from build123d import *

# Parameters (mm, degrees)
SKETCH1_R             = 2
SKETCH1_R_2           = 1.25
BOSS_EXTRUDE1_DEPTH   = 6.1
BOSS_EXTRUDE1_2_DEPTH = 6.1
BOSS_EXTRUDE1_3_DEPTH = 6.1
BOSS_EXTRUDE2_DEPTH   = 1
CUT_EXTRUDE1_REACH    = 18.114
SKETCH6_R             = 1.25


with BuildPart() as part:
    # Sketch1 → Boss-Extrude1 (new body)
    with BuildSketch(Plane.XY):
        with Locations((4, 3.947606604)):
            Circle(SKETCH1_R)
        with Locations((4, 3.947606604)):
            Circle(SKETCH1_R_2, mode=Mode.SUBTRACT)
    extrude(amount=BOSS_EXTRUDE1_DEPTH)



with BuildPart() as body_2:
    # Sketch1 → Boss-Extrude1 2 (new body)
    with BuildSketch(Plane.XY):
        with Locations(Location((-4, 3.947606604, 0), (0, 0, 180))):
            Circle(SKETCH1_R)
        with Locations(Location((-4, 3.947606604, 0), (0, 0, 180))):
            Circle(SKETCH1_R_2, mode=Mode.SUBTRACT)
    extrude(amount=BOSS_EXTRUDE1_2_DEPTH)


with BuildPart() as body_3:
    # Sketch1 → Boss-Extrude1 3 (new body)
    with BuildSketch(Plane.XY):
        with BuildLine():
            Line((7.350565553, 4.525283395), (10.814667168, 6.525283395))
            Line((10.814667168, 6.525283395), (11.414667168, 5.486052911))
            Line((11.414667168, 5.486052911), (8.599175725, 3.860528168))
            ThreePointArc((8.599175725, 3.860528168), (5.132583975, -0.510784758), (0, 1.676043266))
            ThreePointArc((0, 1.676043266), (-5.132583975, -0.510784758), (-8.599175725, 3.860528168))
            Line((-8.599175725, 3.860528168), (-11.414667168, 5.486052911))
            Line((-11.414667168, 5.486052911), (-10.814667168, 6.525283395))
            Line((-10.814667168, 6.525283395), (-7.350565553, 4.525283395))
            ThreePointArc((-7.350565553, 4.525283395), (-1.055513627, 2.247606604), (-6.175565553, 6.560443094))
            Line((-6.175565553, 6.560443094), (-9.639667168, 8.560443094))
            Line((-9.639667168, 8.560443094), (-9.039667168, 9.599673579))
            Line((-9.039667168, 9.599673579), (-6.224175725, 7.974148836))
            ThreePointArc((-6.224175725, 7.974148836), (-2.751650813, 8.374978771), (0, 6.219169942))
            ThreePointArc((0, 6.219169942), (2.751650813, 8.374978771), (6.224175725, 7.974148836))
            Line((6.224175725, 7.974148836), (9.039667168, 9.599673579))
            Line((9.039667168, 9.599673579), (9.639667168, 8.560443094))
            Line((9.639667168, 8.560443094), (6.175565553, 6.560443094))
            ThreePointArc((6.175565553, 6.560443094), (1.055513627, 2.247606604), (7.350565553, 4.525283395))
        make_face()
    extrude(amount=BOSS_EXTRUDE1_3_DEPTH)


with BuildPart() as part_1:
    add(part.part)

    add(body_2.part)  # Boss-Extrude2 merges body 2

    add(body_3.part)  # Boss-Extrude2 merges body 3
    # Sketch2 → Boss-Extrude2 (add)
    with BuildSketch(Plane(origin=(0, 0, 0), x_dir=(-1, 0, 0), z_dir=(0, 0, -1))):
        with BuildLine():
            Line((-9.639667168, 8.560443094), (-10.814667168, 6.525283395))
            Line((-10.814667168, 6.525283395), (-11.414667168, 5.486052911))
            Line((-11.414667168, 5.486052911), (-8.599175725, 3.860528168))
            ThreePointArc((-8.599175725, 3.860528168), (-5.132583975, -0.510784758), (0, 1.676043266))
            ThreePointArc((0, 1.676043266), (5.132583975, -0.510784758), (8.599175725, 3.860528168))
            Line((8.599175725, 3.860528168), (11.414667168, 5.486052911))
            Line((11.414667168, 5.486052911), (10.814667168, 6.525283395))
            Line((10.814667168, 6.525283395), (9.639667168, 8.560443094))
            Line((9.639667168, 8.560443094), (9.039667168, 9.599673579))
            Line((9.039667168, 9.599673579), (6.224175725, 7.974148836))
            ThreePointArc((6.224175725, 7.974148836), (2.751650813, 8.374978771), (0, 6.219169942))
            ThreePointArc((0, 6.219169942), (-2.751650813, 8.374978771), (-6.224175725, 7.974148836))
            Line((-6.224175725, 7.974148836), (-9.039667168, 9.599673579))
            Line((-9.039667168, 9.599673579), (-9.639667168, 8.560443094))
        make_face()
    extrude(amount=BOSS_EXTRUDE2_DEPTH)

    # Sketch6 → Cut-Extrude1 (cut, up to next)
    with BuildSketch(Plane.XY, mode=Mode.PRIVATE) as cut_extrude1_sk1:
        with Locations(Location((4, 3.947606604, 0), (0, 0, 180))):
            Circle(SKETCH6_R)
    cut_extrude1_tool1 = extrude(cut_extrude1_sk1.sketch, amount=-CUT_EXTRUDE1_REACH, mode=Mode.PRIVATE) & part_1.part
    # Sketch6 → Cut-Extrude1 (cut, up to next)
    with BuildSketch(Plane.XY, mode=Mode.PRIVATE) as cut_extrude1_sk2:
        with Locations(Location((-4, 3.947606604, 0), (0, 0, 180))):
            Circle(SKETCH6_R)
    cut_extrude1_tool2 = extrude(cut_extrude1_sk2.sketch, amount=-CUT_EXTRUDE1_REACH, mode=Mode.PRIVATE) & part_1.part
    add(cut_extrude1_tool1.solids().sort_by_distance((4, 3.947607, 0))[0], mode=Mode.SUBTRACT)
    add(cut_extrude1_tool2.solids().sort_by_distance((-4, 3.947607, 0))[0], mode=Mode.SUBTRACT)


solid = part_1.part
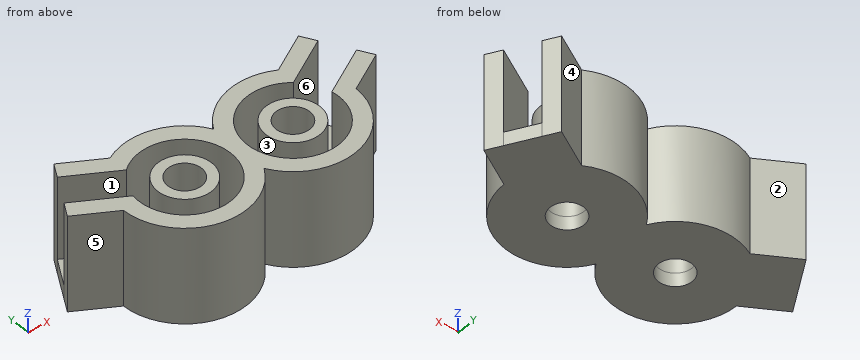
Design review of the part built by this model. Coordinates are the model's own, in mm. Face numbers are marked on the shaded views. A direction names the side the tool comes from. Give positions to 0.01 mm unless a question says otherwise; leave off trailing zeros. Write each loop counter-clockwise with the first axis right and the second up, starting at its lowest first coordinate (ties: lowest second). Pieces come first, ordered by that corner, then holes. Notation, with made-up numbers: M 30,23.5 L 46,23.5 A36 cw 46,57.5 Z; hole C 66.25,26.25 d1. An arc over 180 degrees is marked long. Answer as a JSON object with one key per item and string values. Group by question number.
1) Clearance check with flat-ended pins moving along their axes: pin 1 Ø1.5 at (y, z) = (5.5, 0.5) entering from +X; pin 2 Ø4 at (x, z) = (8, 5) entering from +Y; pin 3 Ø3 at (x, z) = (-7, 3) entering from +Y; pin 4 Ø1 at (x, z) = (7.5, 2.5) entering from +Y. State where each tip first meets the part, or that it passes through.
2) Mouldability with a two-part tool opening along Y and no side actions: class the marked faces 4, 5 and 6 as released by +Y, released by -Y, zero draft, split by the parting line, or undercut.
3) For line 1 along Y through (x, z) = (4, 3); line 2 along X through (y, z) = (1.75, 4); line 3 along Y through (x, z) = (-4, -0.5), list the stretches that pass through material, from the lowest coordinate up.
4) We need section A-A (x = -4). Give the boundary of the cut face in (y, z), and give its area (3 significant figures).
5) Tool access review of the marked faces 1, 2 and 3: name each direction out of +Z, -Z, +X, -X, +Y, -Y from which nothing blocks a thin tool from reaching the whole face with its end or side.
6) We need section B-B (x = -8). Give the boundary of the cut face in (y, z).
Answer key:
{
 "1": {"pin 1": "stops at x = 11.41", "pin 2": "stops at y = 9.6", "pin 3": "stops at y = 9.29", "pin 4": "stops at y = 9"},
 "2": {"face 4": "released by +Y", "face 5": "released by -Y", "face 6": "undercut"},
 "3": {"line 1": "y = -0.65 to 0.55, 1.95 to 2.7, 5.2 to 5.95, 7.35 to 8.55", "line 2": "x = -8.04 to -6.59, -1.41 to 1.41, 6.59 to 8.04", "line 3": "y = -0.65 to 2.7, 5.2 to 8.55"},
 "4": {"outline": "M -0.65,-1 L 2.7,-1 L 2.7,6.1 L 1.95,6.1 L 1.95,0 L 0.55,0 L 0.55,6.1 L -0.65,6.1 Z; M 5.2,-1 L 8.55,-1 L 8.55,6.1 L 7.35,6.1 L 7.35,0 L 5.95,0 L 5.95,6.1 L 5.2,6.1 Z", "area": "30.5 mm²"},
 "5": {"face 1": "+Z, -X", "face 2": "+Z, -Z, +Y", "face 3": "+Z"},
 "6": {"outline": "M 1.68,-1 L 9,-1 L 9,6.1 L 7.61,6.1 L 7.61,0 L 4.9,0 L 4.9,6.1 L 1.68,6.1 Z"}
}
